Autodesk Inventor part; units mm, degrees
ref_plane "Work Plane1" through (0, 0, 6.5) normal (0, 0, 1) x (1, 0, 0)
ref_plane "Work Plane2" through (0, 0, -6.5) normal (0, 0, 1) x (1, 0, 0)
ref_plane "Work Plane3" through (0, 30, 0) normal (0, 1, 0) x (-1, 0, 0)
sketch "Sketch1" plane through (0, 0, 0) normal (0, 0, 1) x (1, 0, 0)
  arc A0 (30, 0) -> (0, 30) centre (0, 0) ccw
  line L0 (30, 0) -> (0, 0)
  line L1 (0, 0) -> (0, 30)
  dimension "d0" = 30
revolve "Revolution1" add sketch "Sketch1" angle 360 about axis through (0, 0, 0) along (0, 1, 0)
sketch "Sketch2" plane through (0, 0, 0) normal (0, 0, 1) x (1, 0, 0)
  circle A0 centre (0, 30) radius 25
  point P0 (0, 0)
  dimension "d2" = 30
  dimension "d3" = 25
extrude "Extrusion1" cut sketch "Sketch2" along normal mid plane 3
ref_plane "Work Plane1" through (0, 0, 6.5) normal (0, 0, 1) x (1, 0, 0)
sketch "Sketch3" plane through (0, 0, 6.5) normal (0, 0, 1) x (1, 0, 0)
  arc A0 (22.7093, 19.5458) -> (-22.7093, 19.5458) centre (0, 0) ccw
  arc A1 (-22.7093, 19.5458) -> (22.7093, 19.5458) centre (0, 30) ccw
extrude "Extrusion2" cut sketch "Sketch3" along normal through all
ref_plane "Work Plane2" through (0, 0, -6.5) normal (0, 0, 1) x (1, 0, 0)
sketch "Sketch4" plane through (0, 0, -6.5) normal (0, 0, 1) x (1, 0, 0)
  arc A0 (22.7093, 19.5458) -> (-22.7093, 19.5458) centre (0, 0) ccw
  arc A1 (-22.7093, 19.5458) -> (22.7093, 19.5458) centre (0, 30) ccw
extrude "Extrusion3" cut sketch "Sketch4" against normal through all
sketch "Sketch5" plane through (0, 0, 6.5) normal (0, 0, 1) x (1, 0, 0)
  line L0 (-30, 0) -> (30, 0)
  point P0 (0, 0)
  point P1 (0, 15)
  dimension "d12" = 15
hole "Hole1" at (0, 15, 6.5) direction (0, 0, -1) diameter 5 end through all
ref_plane "Work Plane3" through (0, 30, 0) normal (0, 1, 0) x (-1, 0, 0)
sketch "Sketch6" plane through (0, 30, 0) normal (0, 1, 0) x (-1, 0, 0)
  line L0 (0, -15) -> (0, 15) construction
  point P0 (0, 0)
  point P1 (0, 0)
  dimension "d21" = 30
hole "Hole2" at (0, 30, -15) at (0, 30, 15) direction (0, -1, 0) diameter 2.5 end through all counterbore diameter 5 counterbore depth 27.5
properties part number "Part004. Spherical Support" material "Steel, Carbon"
Geometry check sheet. Reference: the model listing, model coordinates, mm. A direction names the side the tool comes from. Give positions to 0.01 mm unless a question says otherwise; leave off trailing zeros. Write each loop counter-clockwise with the first axis right and the second up, starting at its lowest first coordinate (ties: lowest second). Pieces come first, ordered by that corner, then holes. Notation, with made-up numbers: M -27.5,-16.5 L 0.5,-16.5 A9 cw 0.5,-7.5 Z; hole C 44.5,87.25 d10. An arc over 180 degrees is marked long. Answer as CSV lines item,"result". Start each with the question number.
Q1. Release check for a two-part mould opening along X. For faces 5 (the face through (0, 5, 18)), 6 (the face through (-0.1, 17.5, -4)), 7 (the face through (0, 0, 0)) record: pulls with the +X half, pulls with the -X half, needs draft (parallel to the pull), parting line crosses it, or undercut.
Q2. Material ranges on L1, parallel to Z at x = 1, y = 5.25; L2, parallel to Z at x = 0, y = 3.85; L3, parallel to Z at x = 0, y = 3.5, recorded low to high.
Q3. Section check A-A, the plane y = 27. Record the cut outline in (x, z).
Q4. Section check D-D, the plane x = 0. Give the number of separate pieces and of enclosed holes in the cut face, then the cut area to 3 significant figures.
Q5. Go/stop test with flat-tipped pins: pin 1 (4 mm diameter, centred on y = 7.5, z = -9.5, fed in from +X); pin 2 (5 mm diameter, centred on x = -10, z = -12, fed in from +Y); pin 3 (12 mm diameter, centred on x = -9.5, z = -14.5, fed in from +Y); pin 4 (3 mm diameter, centred on x = 0, z = 15, fed in from -Y). Record where each tip stops, or that it passes through.
Q6. Tool access check on faces 1 (the face through (-0.1, 17.5, 4)), 2 (the face through (1, 2.5, -16)), 3 (the face through (0, 20, 6.5)), 4 (the face through (0, 5, -18)). Record the directions out of +Z, -Z, +X, -X, +Y, -Y that give a thin tool (end or side, any length) a straight path to the whole face; none if there is none.
Q7. Section check B-B, the plane z = 15. Record the cut outline in (x, y), then the cut area to 3 significant figures.
Q8. Section check C-C, the plane x = 20. Record the cut outline in (y, z), then the cut area to 3 significant figures.
Geometry says:
1,face 5,"undercut"
1,face 6,"undercut"
1,face 7,"needs draft"
2,L1,"-6.5 to -1.5, 1.5 to 6.5"
2,L2,"-29.75 to -17.5, -12.5 to 12.5, 17.5 to 29.75"
2,L3,"-29.8 to -17.5, -12.5 to 12.5, 17.5 to 29.8"
3,outline,"M -12.99,-1.5 A13.08 ccw -11.35,-6.5 L 11.35,-6.5 A13.08 ccw 12.99,-1.5 Z; M -12.99,1.5 L 12.99,1.5 A13.08 ccw 11.35,6.5 L -11.35,6.5 A13.08 ccw Z"
4,separate pieces,"5"
4,enclosed holes,"0"
4,area,"458 mm^2"
5,pin 1,"x = 28.25"
5,pin 2,"y = 8.35"
5,pin 3,"y = 10.38"
5,pin 4,"y = 0"
6,face 1,"+Z, -Z"
6,face 2,"+Y"
6,face 3,"+Z, +Y"
6,face 4,"-Z, +Y"
7,outline,"M -25.98,0 L -1.25,0 L -1.25,2.5 L -2.5,2.5 L -2.5,5.13 A25 cw -20.6,15.83 A25.98 ccw Z; M 1.25,0 L 25.98,0 A25.98 ccw 20.6,15.83 A25 cw 2.5,5.13 L 2.5,2.5 L 1.25,2.5 Z"
7,area,"436 mm^2"
8,outline,"M 0,-22.36 A22.36 ccw 15,-16.58 L 15,-6.5 L 21.4,-6.5 A22.36 ccw 22.31,-1.5 L 15,-1.5 L 15,1.5 L 22.31,1.5 A22.36 ccw 21.4,6.5 L 15,6.5 L 15,16.58 A22.36 ccw 0,22.36 Z"
8,area,"686 mm^2"
